```python
from build123d import *

# Parameters (mm, degrees)
SKETCH3_W           = 20
SKETCH3_H           = 20
BOSS_EXTRUDE1_DEPTH = 300
SKETCH5_W           = 20
SKETCH5_H           = 20
BOSS_EXTRUDE4_DEPTH = 250
SKETCH8_W           = 20
SKETCH8_H           = 20
BOSS_EXTRUDE5_DEPTH = 260
SKETCH13_W          = 230
SKETCH13_H          = 20
BOSS_EXTRUDE7_DEPTH = 20
BOSS_EXTRUDE8_DEPTH = 20
SKETCH15_W          = 20
SKETCH15_H          = 120
BOSS_EXTRUDE9_DEPTH = 20
SKETCH16_R          = 2
CUT_EXTRUDE1_DEPTH  = 20
SKETCH17_R          = 4.2
CUT_EXTRUDE2_DEPTH  = 270
SKETCH19_R          = 1.75
CUT_EXTRUDE3_DEPTH  = 78


with BuildPart() as part:
    # Sketch3 → Boss-Extrude1 (new body)
    with BuildSketch(Plane(origin=(0, 0, 0), x_dir=(1, 0, 0), z_dir=(0, 1, 0))):
        with Locations((10, 10)):
            Rectangle(SKETCH3_W, SKETCH3_H)
    extrude(amount=BOSS_EXTRUDE1_DEPTH)

    # Sketch5 → Boss-Extrude4 (add)
    with BuildSketch(Plane(origin=(0, 0, -20), x_dir=(-1, 0, 0), z_dir=(0, 0, -1))):
        with Locations((-10, 10)):
            Rectangle(SKETCH5_W, SKETCH5_H)
        with Locations((-10, 290)):
            Rectangle(SKETCH5_W, SKETCH5_H)
    extrude(amount=BOSS_EXTRUDE4_DEPTH)

    # Sketch8 → Boss-Extrude5 (add)
    with BuildSketch(Plane(origin=(0, 20, 0), x_dir=(1, 0, 0), z_dir=(0, 1, 0))):
        with Locations((10, 260)):
            Rectangle(SKETCH8_W, SKETCH8_H)
    extrude(amount=BOSS_EXTRUDE5_DEPTH)

    # Sketch13 → Boss-Extrude7 (add)
    with BuildSketch(Plane.ZY):
        with Locations((-135, 50)):
            Rectangle(SKETCH13_W, SKETCH13_H)
    extrude(amount=-BOSS_EXTRUDE7_DEPTH)

    # Sketch14 → Boss-Extrude8 (add)
    with BuildSketch(Plane(origin=(20, 0, 0), x_dir=(0, 0, -1), z_dir=(1, 0, 0))):
        Polygon((125, 200), (20, 200), (20, 180), (125, 180), (145, 180), (250, 180), (250, 200), (145, 200), align=None)
    extrude(amount=-BOSS_EXTRUDE8_DEPTH)

    # Sketch15 → Boss-Extrude9 (add)
    with BuildSketch(Plane(origin=(20, 0, 0), x_dir=(0, 0, -1), z_dir=(1, 0, 0))):
        with Locations((135, 120)):
            Rectangle(SKETCH15_W, SKETCH15_H)
    extrude(amount=-BOSS_EXTRUDE9_DEPTH)

    # Sketch16 → Cut-Extrude1 (cut)
    with BuildSketch(Plane(origin=(20, 0, 0), x_dir=(0, 0, -1), z_dir=(1, 0, 0))):
        with Locations((10, 290)):
            Circle(SKETCH16_R)
        with Locations((10, 190)):
            Circle(SKETCH16_R)
        with Locations((10, 10)):
            Circle(SKETCH16_R)
        with Locations((135, 10)):
            Circle(SKETCH16_R)
        with Locations((135, 290)):
            Circle(SKETCH16_R)
        with Locations(Location((260, 10, 0), (0, 0, 180))):
            Circle(SKETCH16_R)
        with Locations(Location((260, 190, 0), (0, 0, 180))):
            Circle(SKETCH16_R)
        with Locations(Location((260, 290, 0), (0, 0, 180))):
            Circle(SKETCH16_R)
    extrude(amount=-CUT_EXTRUDE1_DEPTH, mode=Mode.SUBTRACT)

    # Sketch17 → Cut-Extrude2 (cut)
    with BuildSketch(Plane(origin=(0, 0, -270), x_dir=(-1, 0, 0), z_dir=(0, 0, -1))):
        with Locations((-10, 10)):
            Circle(SKETCH17_R)
    extrude(amount=-CUT_EXTRUDE2_DEPTH, mode=Mode.SUBTRACT)

    # Sketch19 → Cut-Extrude3 (cut)
    with BuildSketch(Plane(origin=(20, 0, 0), x_dir=(0, 0, -1), z_dir=(1, 0, 0))):
        with Locations((11, 35)):
            Circle(SKETCH19_R)
        with Locations((11, 65)):
            Circle(SKETCH19_R)
        with Locations((259, 35)):
            Circle(SKETCH19_R)
        with Locations((259, 65)):
            Circle(SKETCH19_R)
    extrude(amount=-CUT_EXTRUDE3_DEPTH, mode=Mode.SUBTRACT)


solid = part.part
```
CAD build for the part. Positions are in the model's coordinates, mm. A direction names the side the tool comes from. Give positions to 0.01 mm unless a question says otherwise; leave off trailing zeros. Write each loop counter-clockwise with the first axis right and the second up, starting at its lowest first coordinate (ties: lowest second). Pieces come first, ordered by that corner, then holes. Notation, with made-up numbers: M -32,-2 L 27,-2 A7 ccw 27,8 Z; hole C 49.25,30.5 d1. An arc over 180 degrees is marked long. Return JSON: item names as keys, results as strings. Group by question number.
(1) Band-saw the part on A-A (z = -103.5). Give the cut face in (x, y).
(2) Band-saw the part on B-B (x = 10). State how many separate pieces and enclosed holes the cut face has, and give its area (3 significant figures).
(3) Drill centre lines: L1, parallel to Y at x = 1, z = -47.5; L2, parallel to Z at x = 5.5, y = 190; L3, parallel to Y at x = 8, z = -220.5. Where is each one in solid material? Low to high. Write a range as [from, to].
(4) Band-saw the part on C-C (y = 24). Give the cut face in (x, z), and give its area (3 significant figures).
(5) Mould opens along Y. For faces 1 (the face through (10, 300, -137)), 2 (the face through (10, 280, -133)), 3 (the face through (10, 119, -250)), 4 (the face through (10, 0, -133)) say: pulls with the +Y half, pulls with the -Y half, needs draft (parallel to the pull), parting line crosses it, or undercut.
(6) 3-axis set-ups, long thin cutter, end or side, ignore diameter. For faces 5 (the face through (5.994, 11.262, -136.89)), 6 (the face through (10, 200, -137)): which of +Z, -Z, +X, -X, +Y, -Y reach the whole face in a straight line?
Entries:
{
 "1": {"outline": "M 0,0 L 20,0 L 20,20 L 0,20 Z; M 0,40 L 20,40 L 20,60 L 0,60 Z; M 0,180 L 20,180 L 20,200 L 0,200 Z; M 0,280 L 20,280 L 20,300 L 0,300 Z; hole C 10,10 d8.4"},
 "2": {"separate pieces": "2", "enclosed holes": "13", "area": "30,400 mm^2"},
 "3": {"L1": "y = [0, 20], [40, 60], [180, 200], [280, 300]", "L2": "z = [-270, -262], [-258, -12], [-8, 0]", "L3": "y = [0, 6.31], [13.69, 20], [40, 60], [180, 200], [280, 300]"},
 "4": {"outline": "M 0,-270 L 20,-270 L 20,-250 L 0,-250 Z; M 0,-20 L 20,-20 L 20,0 L 0,0 Z", "area": "800 mm^2"},
 "5": {"face 1": "pulls with the +Y half", "face 2": "undercut", "face 3": "undercut", "face 4": "pulls with the -Y half"},
 "6": {"face 5": "+Z, -Z", "face 6": "+X, -X"}
}
